```python
from build123d import *

# Parameters (mm, degrees)
SKETCH1_R           = 6
BOSS_EXTRUDE1_DEPTH = 10
SKETCH1_7_R         = 23
SKETCH1_7_R_2       = 6
BOSS_EXTRUDE3_DEPTH = 5


with BuildPart() as part:
    # Sketch1 → Boss-Extrude1 (new, symmetric)
    with BuildSketch(Plane.XY):
        Circle(SKETCH1_R)
    extrude(amount=BOSS_EXTRUDE1_DEPTH, both=True)

    # Sketch1<7> → Boss-Extrude3 (add, symmetric)
    with BuildSketch(Plane.XY):
        Circle(SKETCH1_7_R)
        Circle(SKETCH1_7_R_2, mode=Mode.SUBTRACT)
        with BuildLine():
            Line((-1, 14.17544468), (-1, 11.959292144))
            ThreePointArc((-1, 11.959292144), (-1.585786438, 10.545078581), (-3, 9.959292144))
            Line((-3, 9.959292144), (-4.595299462, 9.959292144))
            ThreePointArc((-4.595299462, 9.959292144), (-5.595299462, 9.691342951), (-6.327350269, 8.959292144))
            Line((-6.327350269, 8.959292144), (-7.125, 7.577722283))
            ThreePointArc((-7.125, 7.577722283), (-8.339412717, 6.645870631), (-9.857050808, 6.845671476))
            Line((-9.857050808, 6.845671476), (-11.776295203, 7.953747744))
            ThreePointArc((-11.776295203, 7.953747744), (-12.547269557, 8.756470926), (-12.769788224, 9.846998965))
            ThreePointArc((-12.769788224, 9.846998965), (-12.914018091, 11.506667717), (-13.595491338, 13.02683114))
            ThreePointArc((-13.595491338, 13.02683114), (-13.912573816, 14.417625499), (-13.222255731, 15.66594885))
            ThreePointArc((-13.222255731, 15.66594885), (-10.25, 17.753520778), (-6.955981813, 19.283783784))
            ThreePointArc((-6.955981813, 19.283783784), (-5.529743036, 19.257455106), (-4.483821029, 18.287456446))
            ThreePointArc((-4.483821029, 18.287456446), (-3.50805751, 16.937201591), (-2.142857143, 15.982460485))
            ThreePointArc((-2.142857143, 15.982460485), (-1.309691491, 15.244489647), (-1, 14.17544468))
        make_face(mode=Mode.SUBTRACT)
        with BuildLine():
            Line((4.595299462, 9.959292144), (3, 9.959292144))
            ThreePointArc((3, 9.959292144), (1.585786438, 10.545078581), (1, 11.959292144))
            Line((1, 11.959292144), (1, 14.17544468))
            ThreePointArc((1, 14.17544468), (1.309691491, 15.244489647), (2.142857143, 15.982460485))
            ThreePointArc((2.142857143, 15.982460485), (3.50805751, 16.937201591), (4.483821029, 18.287456446))
            ThreePointArc((4.483821029, 18.287456446), (5.529743036, 19.257455106), (6.955981813, 19.283783784))
            ThreePointArc((6.955981813, 19.283783784), (10.25, 17.753520778), (13.222255731, 15.66594885))
            ThreePointArc((13.222255731, 15.66594885), (13.912573816, 14.417625499), (13.595491338, 13.02683114))
            ThreePointArc((13.595491338, 13.02683114), (12.914018091, 11.506667717), (12.769788224, 9.846998965))
            ThreePointArc((12.769788224, 9.846998965), (12.547269557, 8.756470926), (11.776295203, 7.953747744))
            Line((11.776295203, 7.953747744), (9.857050808, 6.845671476))
            ThreePointArc((9.857050808, 6.845671476), (8.339412717, 6.645870631), (7.125, 7.577722283))
            Line((7.125, 7.577722283), (6.327350269, 8.959292144))
            ThreePointArc((6.327350269, 8.959292144), (5.595299462, 9.691342951), (4.595299462, 9.959292144))
        make_face(mode=Mode.SUBTRACT)
        with BuildLine():
            Line((-10.922649731, -1), (-10.125, -2.38156986))
            ThreePointArc((-10.125, -2.38156986), (-9.925199155, -3.899207951), (-10.857050808, -5.113620668))
            Line((-10.857050808, -5.113620668), (-12.776295203, -6.221696936))
            ThreePointArc((-12.776295203, -6.221696936), (-13.856961048, -6.488018722), (-14.912645367, -6.13546152))
            ThreePointArc((-14.912645367, -6.13546152), (-16.422075601, -5.430533874), (-18.079312367, -5.260625306))
            ThreePointArc((-18.079312367, -5.260625306), (-19.442316853, -4.839829607), (-20.178237544, -3.617834934))
            ThreePointArc((-20.178237544, -3.617834934), (-20.5, 0), (-20.178237544, 3.617834934))
            ThreePointArc((-20.178237544, 3.617834934), (-19.442316853, 4.839829607), (-18.079312367, 5.260625306))
            ThreePointArc((-18.079312367, 5.260625306), (-16.422075601, 5.430533874), (-14.912645367, 6.13546152))
            ThreePointArc((-14.912645367, 6.13546152), (-13.856961048, 6.488018722), (-12.776295203, 6.221696936))
            Line((-12.776295203, 6.221696936), (-10.857050808, 5.113620668))
            ThreePointArc((-10.857050808, 5.113620668), (-9.925199155, 3.899207951), (-10.125, 2.38156986))
            Line((-10.125, 2.38156986), (-10.922649731, 1))
            ThreePointArc((-10.922649731, 1), (-11.190598923, 0), (-10.922649731, -1))
        make_face(mode=Mode.SUBTRACT)
        with BuildLine():
            Line((-4.595299462, -9.959292144), (-3, -9.959292144))
            ThreePointArc((-3, -9.959292144), (-1.585786438, -10.545078581), (-1, -11.959292144))
            Line((-1, -11.959292144), (-1, -14.17544468))
            ThreePointArc((-1, -14.17544468), (-1.309691491, -15.244489647), (-2.142857143, -15.982460485))
            ThreePointArc((-2.142857143, -15.982460485), (-3.50805751, -16.937201591), (-4.483821029, -18.287456446))
            ThreePointArc((-4.483821029, -18.287456446), (-5.529743036, -19.257455106), (-6.955981813, -19.283783784))
            ThreePointArc((-6.955981813, -19.283783784), (-10.25, -17.753520778), (-13.222255731, -15.66594885))
            ThreePointArc((-13.222255731, -15.66594885), (-13.912573816, -14.417625499), (-13.595491338, -13.02683114))
            ThreePointArc((-13.595491338, -13.02683114), (-12.914018091, -11.506667717), (-12.769788224, -9.846998965))
            ThreePointArc((-12.769788224, -9.846998965), (-12.547269557, -8.756470926), (-11.776295203, -7.953747744))
            Line((-11.776295203, -7.953747744), (-9.857050808, -6.845671476))
            ThreePointArc((-9.857050808, -6.845671476), (-8.339412717, -6.645870631), (-7.125, -7.577722283))
            Line((-7.125, -7.577722283), (-6.327350269, -8.959292144))
            ThreePointArc((-6.327350269, -8.959292144), (-5.595299462, -9.691342951), (-4.595299462, -9.959292144))
        make_face(mode=Mode.SUBTRACT)
        with BuildLine():
            Line((6.327350269, -8.959292144), (7.125, -7.577722283))
            ThreePointArc((7.125, -7.577722283), (8.339412717, -6.645870631), (9.857050808, -6.845671476))
            Line((9.857050808, -6.845671476), (11.776295203, -7.953747744))
            ThreePointArc((11.776295203, -7.953747744), (12.547269557, -8.756470926), (12.769788224, -9.846998965))
            ThreePointArc((12.769788224, -9.846998965), (12.914018091, -11.506667717), (13.595491338, -13.02683114))
            ThreePointArc((13.595491338, -13.02683114), (13.912573816, -14.417625499), (13.222255731, -15.66594885))
            ThreePointArc((13.222255731, -15.66594885), (10.25, -17.753520778), (6.955981813, -19.283783784))
            ThreePointArc((6.955981813, -19.283783784), (5.529743036, -19.257455106), (4.483821029, -18.287456446))
            ThreePointArc((4.483821029, -18.287456446), (3.50805751, -16.937201591), (2.142857143, -15.982460485))
            ThreePointArc((2.142857143, -15.982460485), (1.309691491, -15.244489647), (1, -14.17544468))
            Line((1, -14.17544468), (1, -11.959292144))
            ThreePointArc((1, -11.959292144), (1.585786438, -10.545078581), (3, -9.959292144))
            Line((3, -9.959292144), (4.595299462, -9.959292144))
            ThreePointArc((4.595299462, -9.959292144), (5.595299462, -9.691342951), (6.327350269, -8.959292144))
        make_face(mode=Mode.SUBTRACT)
        with BuildLine():
            Line((10.922649731, 1), (10.125, 2.38156986))
            ThreePointArc((10.125, 2.38156986), (9.925199155, 3.899207951), (10.857050808, 5.113620668))
            Line((10.857050808, 5.113620668), (12.776295203, 6.221696936))
            ThreePointArc((12.776295203, 6.221696936), (13.856961048, 6.488018722), (14.912645367, 6.13546152))
            ThreePointArc((14.912645367, 6.13546152), (16.422075601, 5.430533874), (18.079312367, 5.260625306))
            ThreePointArc((18.079312367, 5.260625306), (19.442316853, 4.839829607), (20.178237544, 3.617834934))
            ThreePointArc((20.178237544, 3.617834934), (20.5, 0), (20.178237544, -3.617834934))
            ThreePointArc((20.178237544, -3.617834934), (19.442316853, -4.839829607), (18.079312367, -5.260625306))
            ThreePointArc((18.079312367, -5.260625306), (16.422075601, -5.430533874), (14.912645367, -6.13546152))
            ThreePointArc((14.912645367, -6.13546152), (13.856961048, -6.488018722), (12.776295203, -6.221696936))
            Line((12.776295203, -6.221696936), (10.857050808, -5.113620668))
            ThreePointArc((10.857050808, -5.113620668), (9.925199155, -3.899207951), (10.125, -2.38156986))
            Line((10.125, -2.38156986), (10.922649731, -1))
            ThreePointArc((10.922649731, -1), (11.190598923, 0), (10.922649731, 1))
        make_face(mode=Mode.SUBTRACT)
    extrude(amount=BOSS_EXTRUDE3_DEPTH, both=True)


solid = part.part
```
Could you check a few things on this model? Use its own coordinates, in mm. Round coordinates to 2 decimals unless told otherwise and drop trailing zeros. Order: outer loops, then holes, each group sorted by start corner. A loop starts at its lowest first (then second) coordinate and runs counter-clockwise, first axis right, second up. Notation, with made-up numbers: M 75.25,50.25 L 102.25,50.25 A9 cw 102.25,61.25 Z; hole C 36,35.25 d9. An arc over 180 degrees is marked long. One line per question, with ' | ' between items. Start each with the question number.
(1) Suppose I cut it at D-D on z = -6.75. List the corners of the cut face in (x, y) for me.
(2) Suppose I cut it at B-B on x = 16. List the corners of the cut face in (y, z) for me, then the cut area to 3 significant figures.
(3) Suppose I cut it at A-A on y = 0. List the corners of the cut face in (x, z) for me, then the cut area to 3 significant figures.
(4) Please list where these lines run through material, in increasing order: line 1 along X through (y, z) = (-15.5, 0.75); line 2 along Y through (x, z) = (2, 4.5); line 3 along Y through (x, z) = (-6, 2).
(5) For P1, Ø1, axis at x = -1.5, y = 16.5, coming from the +Z side; P2, Ø0.7, axis at y = -13, z = -1.5, coming from the -X side; P3, Ø1, axis at x = 3, z = -3, coming from the -Y side, each with a flat end and sliding along its axis, tell me the tip position at first contact or that it passes through.
(6) Suppose I cut it at C-C on x = 0. List the corners of the cut face in (y, z) for me, then the cut area to 3 significant figures.
Geometry results:
1) outline: C 0,0 d12
2) outline: M -16.52,-5 L -5.57,-5 L -5.57,5 L -16.52,5 Z; M 5.57,-5 L 16.52,-5 L 16.52,5 L 5.57,5 Z | area: 219 mm²
3) outline: M -23,-5 L -20.5,-5 L -20.5,5 L -23,5 Z; M -11.19,-5 L -6,-5 L -6,-10 L 6,-10 L 6,-5 L 11.19,-5 L 11.19,5 L 6,5 L 6,10 L -6,10 L -6,5 L -11.19,5 Z; M 20.5,-5 L 23,-5 L 23,5 L 20.5,5 Z | area: 394 mm²
4) line 1: -16.99 to -13.4, -1.5 to 1.5, 13.4 to 16.99 | line 2: -22.91 to -15.91, -10.23 to 10.23, 15.91 to 22.91 | line 3: -22.2 to -19.38, -9.38 to 9.38, 19.38 to 22.2
5) P1: z = 5 | P2: x = -19.21 | P3: y = -22.86
6) outline: M -23,-5 L -6,-5 L -6,-10 L 6,-10 L 6,-5 L 23,-5 L 23,5 L 6,5 L 6,10 L -6,10 L -6,5 L -23,5 Z | area: 580 mm²
